Autodesk Inventor part; units mm, degrees
ref_plane "YZ Plane" through (0, 0, 0) normal (1, 0, 0) x (0, 1, 0)
ref_plane "XZ Plane" through (0, 0, 0) normal (0, 1, 0) x (-1, 0, 0)
ref_plane "XY Plane" through (0, 0, 0) normal (0, 0, 1) x (1, 0, 0)
sketch "Sketch1" plane through (0, 0, 0) normal (0, 0, 1) x (1, 0, 0)
  line L0 (0, 0) -> (-25.4, 0)
  line L1 (-25.4, 0) -> (-25.4, 355.6)
  line L2 (-25.4, 355.6) -> (0, 355.6)
  line L3 (0, 355.6) -> (0, 0)
  line L4 (-25.4, 355.6) -> (-273.05, 0)
  line L5 (-273.05, 0) -> (-252.2066, -14.5159)
  line L6 (-252.2066, -14.5159) -> (-4.5566, 341.0841)
  line L7 (-4.5566, 341.0841) -> (-25.4, 355.6)
  point P0 (-25.4, 311.1551)
  dimension "d0" = 25.4
  dimension "d1" = 355.6
  dimension "d2" = 25.4
  dimension "d3" = 273.05
extrude "Extrusion1" add sketch "Sketch1" against normal blind 25.4
sketch "Sketch2" plane through (0, 0, 0) normal (0, 0, 1) x (1, 0, 0)
  line L0 (0, 355.6) -> (0, 0) construction
  line L1 (0, 0) -> (-25.4, 0) construction
  line L2 (-25.4, 0) -> (-25.4, 311.1551) construction
  line L3 (-25.4, 311.1551) -> (-252.2066, -14.5159) construction
  line L4 (-252.2066, -14.5159) -> (-273.05, 0) construction
  line L5 (-273.05, 0) -> (-25.4, 355.6) construction
  line L6 (-25.4, 355.6) -> (0, 355.6) construction
  point P0 (-12.7, 342.9)
  dimension "d6" = 12.7
  dimension "d7" = 12.7
hole "Hole1" at (-12.7, 342.9, 0) direction (0, 0, -1) diameter 5.1054 end through all
equation "\"d2\" = d0"
properties part number "CL6-P1" material "Aluminum 6061"
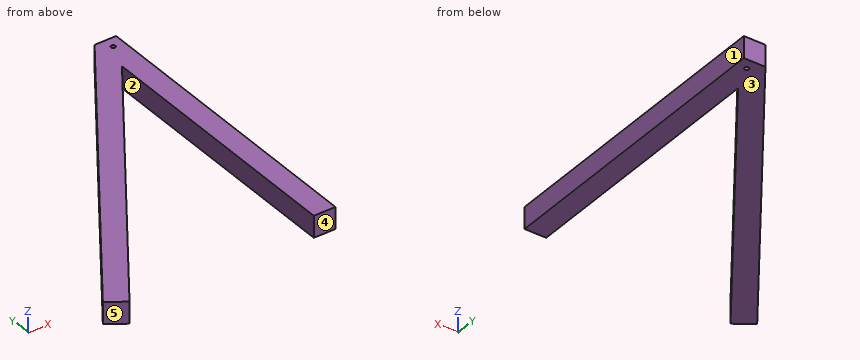
CAD build for the part. Positions are in the model's coordinates, mm. Face numbers are marked on the shaded views. A direction names the side the tool comes from. Coordinates: 2 decimals unless noted, no trailing zeros. Loops run counter-clockwise (first coordinate to the right, second up) from the corner with the lowest first, then second, coordinate; pieces in that order, holes last. Notation, with made-up numbers: (36, -24) - (48, -24) arc R24 ccw to (48, -11) - close; hole circle Ø7 at (88, 37.25). An arc over 180 degrees is marked (long way). Write item = value, one per line. Start each with the question number.
Q1. Drill centre lines: L1, parallel to Y at x = -12.7, z = -9.5; L2, parallel to X at y = 342.9, z = -14.5; L3, parallel to X at y = 70.5, z = -6. Where is each one in solid material? Low to high.
Q2. Cut at C-C, the plane y = 318.5. List the corners of the cut face in (x, z), then the cut area to 3 significant figures.
Q3. Pull direction X, two halves, no side cores. Call the marked faces 1, 2 and 3: pulls with the +X half, pulls with the -X half, needs draft (parallel to the pull), parting line crosses it, or undercut.
Q4. Which spindle directions (+Z, -Z, +X, -X, +Y, -Y) get a long thin tool onto all of the face, cutting with end or side? Do the marked faces 4 and 5. Say none if no direction does.
Q5. Cut at A-A, the plane z = -8.25. List the corners of the cut face in (x, y).
Q6. Flat gauge pins, fed straight in: pin 1 Ø2 at (y, z) = (147.5, -16) entering from -X; pin 2 Ø8 at (x, z) = (-232.5, -4) entering from +Y; pin 3 Ø1.5 at (y, z) = (85, -8.5) entering from -X. Where does each tip first touch, or does it go through?
Q7. Cut at B-B, the plane y = 87. List the corners of the cut face in (x, z), then the cut area to 3 significant figures.
Computed:
q1.L1 = 0 to 340.35, 345.45 to 355.6
q1.L2 = -34.24 to -15.25, -10.15 to 0
q1.L3 = -223.95 to -193, -25.4 to 0
q2.outline = (-51.24, -25.4) - (0, -25.4) - (0, 0) - (-51.24, 0) - close
q2.area = 1,300 mm²
q3.face_1 = pulls with the +X half
q3.face_2 = undercut
q3.face_3 = needs draft
q4.face_4 = +Z, -Z, +X, -Y
q4.face_5 = +Z, -Z, -X, -Y
q5.outline = (-273.05, 0) - (-252.21, -14.52) - (-25.4, 311.16) - (-25.4, 0) - (0, 0) - (0, 355.6) - (-25.4, 355.6) - close; hole circle Ø5.11 at (-12.7, 342.9)
q6.pin_1 = -171.02
q6.pin_2 = 63.97
q6.pin_3 = -214.38
q7.outline = (-212.46, -25.4) - (-181.51, -25.4) - (-181.51, 0) - (-212.46, 0) - close; (-25.4, -25.4) - (0, -25.4) - (0, 0) - (-25.4, 0) - close
q7.area = 1,430 mm²
